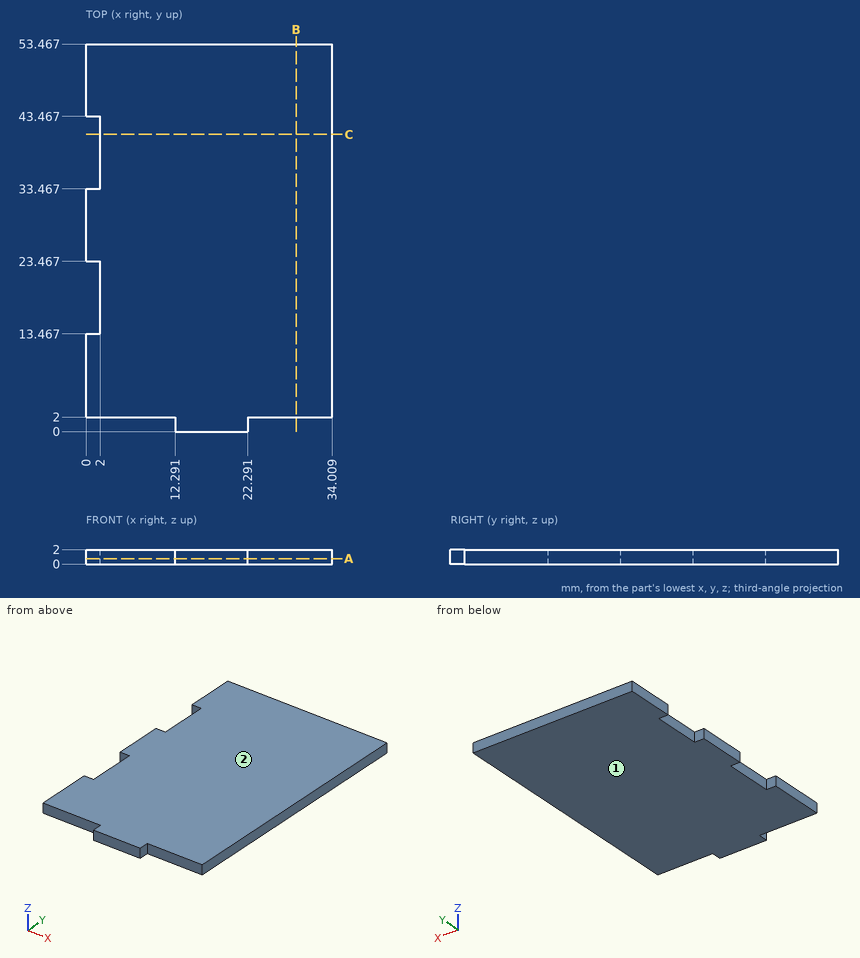
Answer from the drawing. Dimensions are ordinates in mm from the lowest x, y and z of the part. Coordinates: 2 decimals unless noted, no trailing zeros. Write each loop counter-clockwise with the first axis right and the second up, starting at its lowest first coordinate (ties: lowest second). Pieces come first, ordered by that corner, then holes. Notation, with made-up numbers: M -31,55 L 4,55 A17 cw 4,69 Z; hole C 15,32.5 d4. An arc over 180 degrees is marked long. Use one line per item in the form item = value. Start each with the question number.
1. The part is cut by section A-A (z = 0.75). Give the vertices of the cut face in (x, y).
2. Straight lines are drawn through the part: probe 1 along Y at (x, z) = (24.5, 1.65); probe 2 along X at (y, z) = (22.5, 0.25). For each, find the intervals that lie inside material, in ascending order. Write a range as from..to.
3. The mould has two halves that part along Z. Classify the marked faces 1 and 2: released by +Z, released by -Z, zero draft, split by the parting line, or undercut.
4. The part is cut by section B-B (x = 29). Give the vertices of the cut face in (y, z), plus the area to 3 significant figures.
5. Each of these flat-tipped pins is pushed along its axis until it touches: P1, Ø1, axis at x = 0.5, z = 0.5, coming from the -Y side; P2, Ø0.6, axis at y = 16, z = 1, coming from the -X side; P3, Ø1, axis at y = 1, z = 0.5, coming from the -X side. Where does it stop, or does it pass through?
6. The part is cut by section C-C (y = 41). Give the vertices of the cut face in (x, z).
Evaluation:
q1.outline = M 0,2 L 12.29,2 L 12.29,0 L 22.29,0 L 22.29,2 L 34.01,2 L 34.01,53.47 L 0,53.47 L 0,43.47 L 2,43.47 L 2,33.47 L 0,33.47 L 0,23.47 L 2,23.47 L 2,13.47 L 0,13.47 Z
q2.probe_1 = 2..53.47
q2.probe_2 = 2..34.01
q3.face_1 = released by -Z
q3.face_2 = released by +Z
q4.outline = M 2,0 L 53.47,0 L 53.47,2 L 2,2 Z
q4.area = 103 mm^2
q5.P1 = 2
q5.P2 = 2
q5.P3 = 12.29
q6.outline = M 2,0 L 34.01,0 L 34.01,2 L 2,2 Z
